Input: part model. Units: mm. Frame: model coordinates. A direction names the side the tool comes from. Coordinates: 2 decimals unless noted, no trailing zeros. Order: outer loops, then holes, each group sorted by start corner. A loop starts at its lowest first (then second) coordinate and runs counter-clockwise, first axis right, second up. Notation, with made-up numbers: (47.25, 57.25) - (105.25, 57.25) arc R25 cw to (105.25, 91.25) - close; hole circle Ø5 at (-9, 28.25). An arc over 180 degrees is marked (long way). One line per question, with ' | ' between items.
from build123d import *

# Parameters (mm, degrees)
SKETCH_3_R      = 1.5
EXTRUDE_1_DEPTH = 1.7


with BuildPart() as part:
    # Эскиз3 → Бобышка-Вытянуть1 (new body)
    with BuildSketch(Plane.XY):
        with BuildLine():
            Line((-6.473729419, -32.810303411), (-6.068906589, -30.772625658))
            ThreePointArc((-6.068906589, -30.772625658), (-7.567661229, -26.882580179), (-11.724624303, -26.568928632))
            ThreePointArc((-11.724624303, -26.568928632), (-14.962869732, -27.255997351), (-18.072620871, -26.12120894))
            ThreePointArc((-18.072620871, -26.12120894), (0, 29.4), (18.072620871, -26.12120894))
            ThreePointArc((18.072620871, -26.12120894), (14.962869732, -27.255997351), (11.724624303, -26.568928632))
            ThreePointArc((11.724624303, -26.568928632), (7.567661229, -26.882580179), (6.068906589, -30.772625658))
            Line((6.068906589, -30.772625658), (6.473729419, -32.810303411))
            ThreePointArc((6.473729419, -32.810303411), (7.37290154, -34.115019127), (8.938996834, -34.356139707))
            ThreePointArc((8.938996834, -34.356139707), (0, 35.5), (-8.938996834, -34.356139707))
            ThreePointArc((-8.938996834, -34.356139707), (-7.37290154, -34.115019127), (-6.473729419, -32.810303411))
        make_face()
        with Locations((-9.89414741, -30.012669962)):
            Circle(SKETCH_3_R, mode=Mode.SUBTRACT)
        with Locations(Location((9.89414741, -30.012669962, 0), (0, 0, 180))):
            Circle(SKETCH_3_R, mode=Mode.SUBTRACT)
    extrude(amount=EXTRUDE_1_DEPTH)


solid = part.part
Item 1: Ray query, line 1 (X direction, y = -16.5, z = 1.65); line 2 (X direction, y = -22, z = 0.2); line 3 (Y direction, x = 22, z = 1.55). Return the intervals inside material, ascending.
Data:
line 1: -31.43 to -26.68, 26.68 to 31.43 | line 2: -27.86 to -22.68, 22.68 to 27.86 | line 3: -27.86 to -22.72, 20.11 to 27.86
Item 2: Section B-B on y = 14. Return the cut outline in (x, z), and give its area (3 significant figures).
Data:
outline: (-32.62, 0) - (-26.62, 0) - (-26.62, 1.7) - (-32.62, 1.7) - close; (26.62, 0) - (32.62, 0) - (32.62, 1.7) - (26.62, 1.7) - close | area: 20.4 mm^2
Item 3: Section A-A on x = -19.5. Return the cut outline in (y, z).
Data:
outline: (-29.66, 0) - (-25.02, 0) - (-25.02, 1.7) - (-29.66, 1.7) - close; (22.41, 0) - (29.66, 0) - (29.66, 1.7) - (22.41, 1.7) - close
Item 4: Draft query along Y for faces 4 (the face through (5.1, 29.2, 0)), 5 (the face through (1.43, 35.47, 0.84)), 6 (the face through (-14.92, -27.26, 0.84)), 7 (the face through (-6.274, -31.806, 0.838)). Return one class per face: released by +Y, released by -Y, zero draft, split by the parting line, or undercut.
Data:
face 4: zero draft | face 5: split by the parting line | face 6: undercut | face 7: released by -Y
Item 5: Contact query for flat-ended pins moving along their axis: P1, Ø1.8, axis at x = -9.89, y = -30.01, coming from the +Z side; P2, Ø1, axis at x = -22, z = 1, coming from the +Y side. Output: stop coordinate, or through.
Data:
P1: through | P2: y = 28.25
Item 6: Section C-C on z = 1. Return the cut outline in (x, y).
Data:
outline: (-18.07, -26.12) arc R30.7 cw (long way) to (18.07, -26.12) arc R6 cw to (11.72, -26.57) arc R3.9 ccw to (6.07, -30.77) - (6.47, -32.81) arc R2 ccw to (8.94, -34.36) arc R35.5 ccw (long way) to (-8.94, -34.36) arc R2 ccw to (-6.47, -32.81) - (-6.07, -30.77) arc R3.9 ccw to (-11.72, -26.57) arc R6 cw to start; hole circle Ø3 at (-9.89, -30.01); hole circle Ø3 at (9.89, -30.01)
Item 7: Section D-D on x = 0. Return the cut outline in (y, z), and give its area (3 significant figures).
Data:
outline: (29.4, 0) - (35.5, 0) - (35.5, 1.7) - (29.4, 1.7) - close | area: 10.4 mm^2
Item 8: Access query for faces 1 (the face through (6.27, -31.78, 0.84)), 2 (the face through (15.01, -27.253, 0.838)), 3 (the face through (5.1, 29.2, 1.7)). Directions: +Z, -Z, +X, -X, +Y, -Y. A direction counts if a zero-diameter tool reaches every point of the face in a straight line with its end or side. Return the directions, or none.
Data:
face 1: +Z, -Z, -Y | face 2: +Z, -Z | face 3: +Z, +X, -X, +Y, -Y
